The listing builds one solid part. Answer for the finished solid, in the listing's coordinates (mm). Coordinates: 2 decimals unless noted, no trailing zeros. Order: outer loops, then holes, each group sorted by start corner. A loop starts at its lowest first (then second) coordinate and runs counter-clockwise, first axis right, second up. Notation, with made-up numbers: (-37.5, 61) -> (7.5, 61) arc R16 ccw to (7.5, 91) -> close; hole circle Ø8 at (71.25, 76). An arc over 180 degrees is marked (long way). Return JSON: item names as keys, results as strings.
```python
from build123d import *

# Parameters (mm, degrees)
SKETCH1_W           = 50
SKETCH1_H           = 80
SKETCH1_R           = 4.5
BOSS_EXTRUDE1_DEPTH = 25
SKETCH2_R           = 6
CUT_EXTRUDE1_DEPTH  = 81
CHAMFER1_SIZE       = 1


with BuildPart() as part:
    # Sketch1 → Boss-Extrude1 (new body)
    with BuildSketch(Plane(origin=(0, 0, 0), x_dir=(1, 0, 0), z_dir=(0, 1, 0))):
        Rectangle(SKETCH1_W, SKETCH1_H)
        with Locations((15.5, 24.8)):
            Circle(SKETCH1_R, mode=Mode.SUBTRACT)
        with Locations((-15.5, -24.8)):
            Circle(SKETCH1_R, mode=Mode.SUBTRACT)
    extrude(amount=BOSS_EXTRUDE1_DEPTH)

    # Sketch2 → Cut-Extrude1 (cut, through all)
    with BuildSketch(Plane.XY.offset(40)):
        with Locations((0, 12.5)):
            Circle(SKETCH2_R)
    extrude(amount=-CUT_EXTRUDE1_DEPTH, mode=Mode.SUBTRACT)

    # Chamfer1
    chamfer1_edges = [part.edges().sort_by_distance(p)[0] for p in [
        (11, 0, -24.8),
        (11, 25, -24.8),
        (-20, 0, 24.8),
        (-20, 25, 24.8),
        (-6, 12.5, -40),
        (-6, 12.5, 40),
    ]]
    chamfer(chamfer1_edges, length=CHAMFER1_SIZE)


solid = part.part
```
Item 1: Determine the mould class of faces 1 (the flat face through (-25, 12, 1)), 2 (the cylindrical face through (-19.1, 12.3, 27.5)), 3 (the flat face through (-6, 7, 40)) for opening direction Z: pulls with the +Z half, pulls with the -Z half, needs draft (parallel to the pull), parting line crosses it, or undercut.
Answer list:
{"face 1": "needs draft", "face 2": "undercut", "face 3": "pulls with the +Z half"}
Item 2: The part is cut by section B-B on z = -24.8. Determine the outline of the cut face in (x, y).
Answer list:
{"outline": "(-25, 0) -> (10, 0) -> (11, 1) -> (11, 24) -> (10, 25) -> (-25, 25) -> close; (20, 1) -> (21, 0) -> (25, 0) -> (25, 25) -> (21, 25) -> (20, 24) -> close; hole circle Ø12 at (0, 12.5)"}
Item 3: Find the intervals of material crossed by probe 1 along Z at (x, y) = (-15.5, 11.75); probe 2 along X at (y, z) = (16, 24.8); probe 3 along X at (y, z) = (12.25, 10.5), in increasing order.
Answer list:
{"probe 1": "-40 to 20.3, 29.3 to 40", "probe 2": "-25 to -20, -11 to -4.87, 4.87 to 25", "probe 3": "-25 to -5.99, 5.99 to 25"}
Item 4: The part is cut by section A-A on y = 12.5. Determine the outline of the cut face in (x, z).
Answer list:
{"outline": "(-25, -40) -> (-7, -40) -> (-6, -39) -> (-6, 39) -> (-7, 40) -> (-25, 40) -> close; (6, -39) -> (7, -40) -> (25, -40) -> (25, 40) -> (7, 40) -> (6, 39) -> close; hole circle Ø9 at (-15.5, 24.8); hole circle Ø9 at (15.5, -24.8)"}
Item 5: The part is cut by section D-D on y = 2.75. Determine the outline of the cut face in (x, z), plus the area to 3 significant figures.
Answer list:
{"outline": "(-25, -40) -> (25, -40) -> (25, 40) -> (-25, 40) -> close; hole circle Ø9 at (-15.5, 24.8); hole circle Ø9 at (15.5, -24.8)", "area": "3,870 mm2"}
Item 6: The part is cut by section C-C on x = 15.5. Determine the outline of the cut face in (y, z).
Answer list:
{"outline": "(0, -40) -> (25, -40) -> (25, -30.3) -> (24, -29.3) -> (1, -29.3) -> (0, -30.3) -> close; (0, -19.3) -> (1, -20.3) -> (24, -20.3) -> (25, -19.3) -> (25, 40) -> (0, 40) -> close"}
